Input: part model. Units: mm. Frame: model coordinates. Give positions to 0.01 mm unless a question says otherwise; leave off trailing zeros. Answer as a JSON object with one key per item and string values.
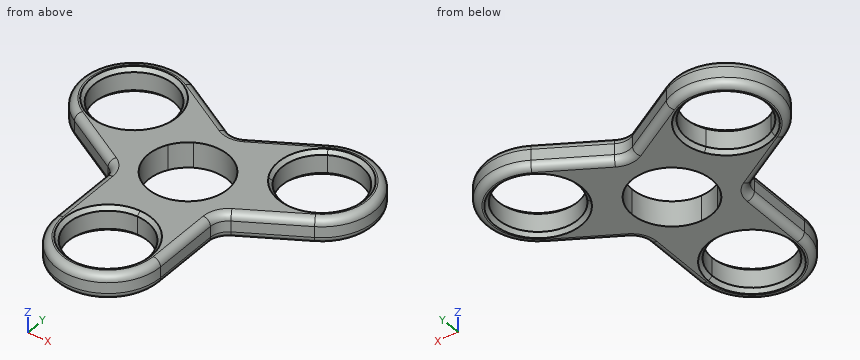
from build123d import *

# Parameters (mm, degrees)
F1_DEPTH    = 7
F3_DEPTH    = 7.001
F5_COUNT    = 3
F7_T1_DEPTH = 7
F8_R        = 2
F9_SIZE     = 1


# Not quite as in the source:
# - a fillet or chamfer that OpenCascade refuses, or shapes differently, is made with other operations: its cross-section is extruded or revolved along the edge and cut away or added
# - a feature names something its author has since deleted; it is built from what else it names


with BuildPart() as f1:
    # F0 (on Top) → F1 (new body)
    with BuildSketch(Plane.XY):
        with BuildLine():
            ThreePointArc((-14.5, 0), (0, -14.5), (14.5, 0))
            ThreePointArc((14.5, 0), (0, 14.5), (-14.5, 0))
        make_face()
        with BuildLine():
            Line((14.5, -30), (14.5, 0))
            ThreePointArc((14.5, 0), (0, -14.5), (-14.5, 0))
            Line((-14.5, 0), (-14.5, -30))
            ThreePointArc((-14.5, -30), (0, -15.5), (14.5, -30))
        make_face()
        with BuildLine():
            ThreePointArc((-14.5, -30), (0, -44.5), (14.5, -30))
            ThreePointArc((14.5, -30), (0, -15.5), (-14.5, -30))
        make_face()
    extrude(amount=F1_DEPTH)

    # F2 (on face) → F3 (cut, through all)
    with BuildSketch(Plane.XY.offset(7)):
        with BuildLine():
            ThreePointArc((0, -11), (7.7781745931, -7.7781745931), (11, 0))
            ThreePointArc((11, 0), (-7.7781745931, 7.7781745931), (0, -11))
        make_face()
        with BuildLine():
            ThreePointArc((11, -30), (7.7781745931, -22.2218254069), (0, -19))
            ThreePointArc((0, -19), (-7.7781745931, -37.7781745931), (11, -30))
        make_face()
    extrude(amount=-F3_DEPTH, mode=Mode.SUBTRACT)


with BuildPart() as f5_1:
    # F5: instance of F1
    add(f1.part.rotate(Axis((0, 0, 13.2415927947), (0, 0, 1)), 1 * 360 / F5_COUNT))


with BuildPart() as f5_2:
    # F5: instance of F1
    add(f1.part.rotate(Axis((0, 0, 13.2415927947), (0, 0, 1)), 2 * 360 / F5_COUNT))


with BuildPart() as f1_1:
    add(f1.part)

    # F6: union F5_2, F5_1
    add(f5_2.part)
    add(f5_1.part)

    # F7: fillet of radius 5 on 6 edges, made by hand

    # F7_s2 → F7_t1 (join)
    with BuildSketch(Plane.XY):
        with BuildLine():
            ThreePointArc((17, -6.9282032303), (15.1698729811, -8.7583302492), (14.5, -11.2583302492))
            Line((14.5, -11.2583302492), (14.5, -8.3715789032))
            Line((14.5, -8.3715789032), (17, -6.9282032303))
        make_face()
        with BuildLine():
            ThreePointArc((-2.5, 18.1865334795), (0, 17.5166604984), (2.5, 18.1865334795))
            Line((2.5, 18.1865334795), (0, 16.7431578065))
            Line((0, 16.7431578065), (-2.5, 18.1865334795))
        make_face()
        with BuildLine():
            ThreePointArc((-14.5, -11.2583302492), (-15.1698729811, -8.7583302492), (-17, -6.9282032303))
            Line((-17, -6.9282032303), (-14.5, -8.3715789032))
            Line((-14.5, -8.3715789032), (-14.5, -11.2583302492))
        make_face()
    extrude(amount=F7_T1_DEPTH)

    # F8
    f8_edges = [f1_1.edges().sort_by_distance(p)[0] for p in [
        (38.53813, 22.25, 7),
        (0, -44.5, 0),
        (-25.115381, -2.242786, 0),
        (-15.169873, -8.75833, 0),
        (-14.5, -20.629165, 0),
        (14.5, -20.629165, 0),
        (15.169873, -8.75833, 0),
        (25.115381, -2.242786, 0),
        (38.53813, 22.25, 0),
        (10.615381, 22.871951, 0),
        (0, 17.51666, 0),
        (-10.615381, 22.871951, 0),
        (-38.53813, 22.25, 0),
        (-25.115381, -2.242786, 7),
        (-14.5, -20.629165, 7),
        (0, -44.5, 7),
        (14.5, -20.629165, 7),
        (25.115381, -2.242786, 7),
        (10.615381, 22.871951, 7),
        (-10.615381, 22.871951, 7),
        (-38.53813, 22.25, 7),
        (-15.169873, -8.75833, 7),
        (15.169873, -8.75833, 7),
        (0, 17.51666, 7),
    ]]
    fillet(f8_edges, radius=F8_R)

    # F9
    f9_edges = [f1_1.edges().sort_by_distance(p)[0] for p in [
        (-35.507042, 20.5, 7),
        (0, -41, 7),
        (35.507042, 20.5, 7),
        (0, -41, 0),
        (35.507042, 20.5, 0),
        (-35.507042, 20.5, 0),
    ]]
    chamfer(f9_edges, length=F9_SIZE)


solid = f1_1.part
Item 1: Cut plane A-A (x = -1). Give the number of separate pieces and of enclosed holes in the cut face, then the cut area to 3 significant figures.
Geometry check:
{"separate pieces": "3", "enclosed holes": "0", "area": "122 mm2"}
Item 2: Material intervals for line 1 (Y direction, x = 0, z = 2.1); line 2 (X direction, y = -30, z = 3.85); line 3 (Y direction, x = 8, z = 3.25), sorted ascending. Write a range as [from, to].
Geometry check:
{"line 1": "y = [-44.5, -41], [-19, -11], [11, 17.52]", "line 2": "x = [-14.5, -11], [11, 14.5]", "line 3": "y = [-42.09, -37.55], [-22.45, -7.55], [7.55, 21.36]"}
Item 3: Contact query for flat-ended pins moving along their axis: P1, Ø12, axis at x = 22, y = -5, coming from the +Z side; P2, Ø3.5, axis at y = -22, z = 4, coming from the +X side; P3, Ø0.9, axis at y = -21, z = 4, coming from the -X side; P4, Ø2, axis at x = 11, z = 3, coming from the -Y side. Output: stop coordinate, or through.
Geometry check:
{"P1": "stops at z = 7", "P2": "stops at x = 14.5", "P3": "stops at x = -14.5", "P4": "stops at y = -40.5"}
